```python
from build123d import *

# Parameters (mm, degrees)
F1_DEPTH = 31.75
F0_R     = 49.2494250879
F2_DEPTH = 25.4
F3_R     = 5.08


with BuildPart() as f1:
    # F0 (on Front) → F1 (new body)
    with BuildSketch(Plane.XZ):
        with BuildLine():
            Line((-40.602091343, 27.9041671834), (-75.195086289, 27.9041671834))
            ThreePointArc((-75.195086289, 27.9041671834), (-64.9651755745, 3.6226405346), (-40.602091343, -6.4114880449))
            Line((-40.602091343, -6.4114880449), (-40.602091343, 27.9041671834))
        make_face()
        with BuildLine():
            Line((-40.602091343, 28.1826276332), (-40.602091343, 62.7767433114))
            ThreePointArc((-40.602091343, 62.7767433114), (-65.1620784416, 52.5457118647), (-75.195086289, 27.9041671834))
            Line((-75.195086289, 27.9041671834), (-40.602091343, 27.9041671834))
            Line((-40.602091343, 27.9041671834), (-40.602091343, 28.1826276332))
        make_face()
        with BuildLine():
            ThreePointArc((-6.0090963971, 27.9041671834), (-6.0082558491, 28.0433962806), (-6.0079756649, 28.1826276332))
            ThreePointArc((-6.0079756649, 28.1826276332), (-16.1403575579, 52.6443614184), (-40.602091343, 62.7767433114))
            Line((-40.602091343, 62.7767433114), (-40.602091343, 28.1826276332))
            Line((-40.602091343, 28.1826276332), (-40.602091343, 27.9041671834))
            Line((-40.602091343, 27.9041671834), (-6.0090963971, 27.9041671834))
        make_face()
        with BuildLine():
            ThreePointArc((-40.602091343, -6.4114880449), (-16.2390071116, 3.6226405346), (-6.0090963971, 27.9041671834))
            Line((-6.0090963971, 27.9041671834), (-40.602091343, 27.9041671834))
            Line((-40.602091343, 27.9041671834), (-40.602091343, -6.4114880449))
        make_face()
    extrude(amount=F1_DEPTH)

    # F0 (on Front) → F2 (join)
    with BuildSketch(Plane.XZ):
        with Locations((-40.602091343, 28.1826276332)):
            Circle(F0_R)
        with BuildLine():
            ThreePointArc((-40.602091343, 62.7767433114), (-16.1403575579, 52.6443614184), (-6.0079756649, 28.1826276332))
            ThreePointArc((-6.0079756649, 28.1826276332), (-6.0082558491, 28.0433962806), (-6.0090963971, 27.9041671834))
            ThreePointArc((-6.0090963971, 27.9041671834), (-16.2390071116, 3.6226405346), (-40.602091343, -6.4114880449))
            ThreePointArc((-40.602091343, -6.4114880449), (-64.9651755745, 3.6226405346), (-75.195086289, 27.9041671834))
            ThreePointArc((-75.195086289, 27.9041671834), (-65.1620784416, 52.5457118647), (-40.602091343, 62.7767433114))
        make_face(mode=Mode.SUBTRACT)
    extrude(amount=F2_DEPTH)

    # F3
    f3_edges = [f1.edges().sort_by_distance(p)[0] for p in [
        (-40.602091, -31.75, 62.776743),
        (-89.851516, -25.4, 28.182628),
    ]]
    fillet(f3_edges, radius=F3_R)


solid = f1.part
```
Part model, mm, in its own coordinate system. A direction names the side the tool comes from. Round coordinates to 2 decimals unless told otherwise and drop trailing zeros. Write each loop counter-clockwise with the first axis right and the second up, starting at its lowest first coordinate (ties: lowest second). Pieces come first, ordered by that corner, then holes. Notation, with made-up numbers: M 52,11.25 L 79,11.25 A21 ccw 79,17.25 Z; hole C -4,40.5 d5. An arc over 180 degrees is marked long. Answer as CSV lines item,"result". Start each with the question number.
1) Drill centre lines: L1, parallel to Z at x = -42, y = -11; L2, parallel to Y at x = -60.5, z = 61.5; L3, parallel to X at y = -16, z = 27.5. Where is each one in solid material? Low to high.
2) Band-saw the part on B-B (y = -23.5). List the corners of the cut face in (x, z).
3) Drop flat-ended pins along their axis: pin 1 (10 mm diameter, centred on x = -46.5, y = -3.5, fed in from -Z); pin 2 (4 mm diameter, centred on y = -26.5, z = 51.5, fed in from -X); pin 3 (1.5 mm diameter, centred on y = -6.5, z = 15, fed in from +X). Give the stop position or say it passes through.
4) Band-saw the part on A-A (y = -17). List the corners of the cut face in (x, z).
5) Which spindle directions (+Z, -Z, +X, -X, +Y, -Y) get a long thin tool onto all of the face, cutting with end or side? Do faces 1 (the face through (-67, -25.4, 5)), 2 (the face through (-41, -31.75, 29)). Say none if no direction does.
Worked out:
1,L1,"-21.05 to 77.41"
1,L2,"-25.4 to 0"
1,L3,"-89.85 to 8.64"
2,outline,"C -40.6,28.18 d96.26"
3,pin 1,"z = -21.06"
3,pin 2,"x = -81.65"
3,pin 3,"x = 7.05"
4,outline,"C -40.6,28.18 d98.5"
5,face 1,"-Y"
5,face 2,"+Z, -Z, +X, -X, -Y"
